Work out the finished part from the listing and answer in its coordinate system (mm). Face numbers are marked on the shaded views. A direction names the side the tool comes from. Coordinates: 2 decimals unless noted, no trailing zeros. Order: outer loops, then holes, each group sorted by start corner. A loop starts at its lowest first (then second) coordinate and runs counter-clockwise, first axis right, second up. Notation, with made-up numbers: (-11.5, -16) -> (16.5, -16) arc R23 ccw to (16.5, 15) -> close; hole circle Ø5 at (30, 9.25). An arc over 180 degrees is marked (long way). Use one line per item in the form item = value.
Autodesk Inventor part; units mm, degrees
ref_plane "Work Plane1" through (1.525, 0, 0) normal (0, 0, 1) x (1, 0, 0)
ref_plane "YZ Plane" through (0, 0, 0) normal (1, 0, 0) x (0, 1, 0)
ref_plane "XZ Plane" through (0, 0, 0) normal (0, 1, 0) x (-1, 0, 0)
sketch "Sketch1" plane through (0, 0, 0) normal (0, 0, 1) x (1, 0, 0)
  line L0 (0, 5.0006) -> (0, 3.175)
  line L1 (3.175, 3.175) -> (19.05, 3.175)
  line L2 (19.05, 3.175) -> (19.05, 0)
  line L3 (19.05, 0) -> (-0.6351, 0)
  line L4 (-4.5721, 0) -> (22.987, 0)
  line L5 (-0.6351, 0) -> (-0.6351, 5.0006)
  line L6 (-0.6351, 5.0006) -> (0, 5.0006)
  line L7 (3.175, 3.175) -> (1.9049, 3.175)
  line L8 (1.9049, 3.175) -> (0, 3.175)
  line L9 (0, -1.0001) -> (0, 6.0007)
  dimension "d0" = 19.05
  dimension "d1" = 15.875
  dimension "d2" = 6.35
  dimension "d9" = 0.6351
  dimension "d10" = 10.0013
  dimension "d13" = 1.2701
  dimension "d14" = 6.35
revolve "Body" add sketch "Sketch1" angle 360 about axis through (19.05, 0, 0) along (-1, 0, 0)
sketch "Sketch2" plane through (-0.6351, 0, 0) normal (-1, 0, 0) x (0, 0, 1)
  line L0 (0, 6.4158) -> (5.5562, 3.2079)
  line L1 (5.5562, 3.2079) -> (5.5562, -3.2079)
  line L2 (5.5562, -3.2079) -> (0, -6.4158)
  line L3 (0, -6.4158) -> (-5.5562, -3.2079)
  line L4 (-5.5562, -3.2079) -> (-5.5562, 3.2079)
  line L5 (-5.5562, 3.2079) -> (0, 6.4158)
  point P0 (0, 0)
  point P1 (0, 0)
  dimension "d11" = 11.1125
extrude "Head" add sketch "Sketch2" along normal blind 3.3337
sketch "Sketch4" plane through (0, 0, 0) normal (0, 0, 1) x (1, 0, 0)
  line L0 (-3.9689, 5.5563) -> (-3.9689, 6.4158)
  line L1 (-3.9689, 6.4158) -> (-3.4726, 6.4158)
  line L2 (-3.4726, 6.4158) -> (-3.9689, 5.5563)
  line L3 (-4.6356, 0) -> (0.0317, 0)
  line L4 (-0.6351, 6.4158) -> (-3.9688, 6.4158)
  line L5 (-3.9688, 3.2079) -> (-3.9688, 6.4158)
  dimension "d5" = 30
  dimension "d19" = 11.1125
revolve "Chamfer1" cut sketch "Sketch4" angle 360 about axis through (-10, 0, 0) along (1, 0, 0)
thread "Thread"
chamfer "Chamfer2" distance 0.6875 distance2 1.2701 1 edges at (19.05, -3.175, 0) measured on face at (19.05, -0.5663, 0.5832)
ref_plane "Work Plane1" through (1.525, 0, 0) normal (0, 0, 1) x (1, 0, 0)
fillet "Fillet2" radius 0.635 1 edges at (0, -3.175, 0)
equation "\"d0\" = NLG"
equation "\"d1\" = GEL"
equation "\"d2\" = GD"
equation "\"d10\" = SD2"
equation "\"d14\" = BDM"
equation "\"d11\" = SW"
equation "\"d3\" = KOH - SD"
equation "\"d5\" = ANG1"
equation "\"d19\" = SW0"
equation "\"d63\" = R"
equation "\"d15\" = GEL"
equation "\"d6\" = -0.5 * SPD + 0.5 * GD"
equation "\"NLG\" = 19.05"
equation "\"GD\" = NND"
equation "\"BDM\" = 6.35"
equation "\"KOH\" = 3.96875"
equation "\"GEL\" = 15.875"
equation "\"SW\" = 11.1125"
equation "\"SW0\" = SW"
equation "\"SPD\" = 4.9751"
equation "\"SD2\" = 10.00125"
equation "\"SD\" = 0.635"
equation "\"ANG1\" = 30deg"
equation "\"GAL\" = 1.27"
equation "\"GUL\" = 1.27"
equation "\"R\" = 0.635"
equation "\"d62\" = -NLG - SD + GUL"
equation "\"THREADDIA\" = 6.35"
equation "\"TOA\" = 30deg"
equation "\"RR\" = 0.254"
equation "\"NND\" = 6.35"
equation "\"E0\" = 1.155 * SW"
equation "\"SLG\" = 0"
equation "\"GD1\" = 4.9751"
properties part number "ANSI B18.2.1 - 1/4-20 UNC - 0.75" material "Steel, Mild"
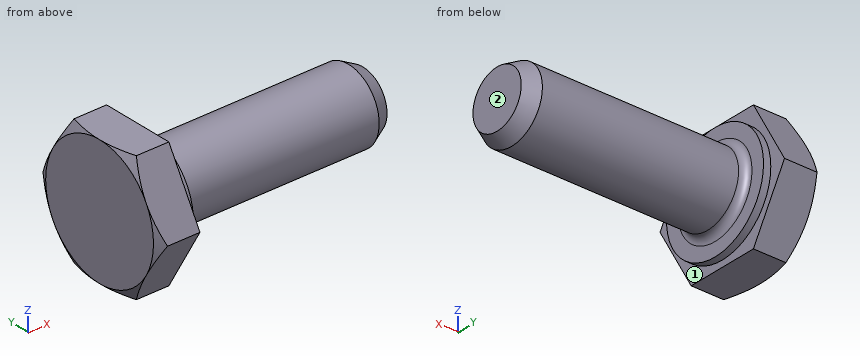
(1) Straight lines are drawn through the part: line 1 along X through (y, z) = (4.75, 1); line 2 along X through (y, z) = (3, 4.25); line 3 along Y through (x, z) = (-2.5, 2.5). For each, find the intervals that lie inside material, in ascending order.
Data:
line_1 = -3.97 to 0
line_2 = -3.97 to -0.64
line_3 = -4.97 to 4.97
(2) Section A-A on x = 5.75 is taken. Write down the section's boundary in (y, z) (3 decimals), plus the area to 3 significant figures.
Data:
outline = circle Ø6.35 at (0, 0)
area = 31.7 mm²
(3) Which of the six approach directions +Z, -Z, +X, -X, +Y, -Y give full straight-line access (tool end or side, diameter ignored) to the marked faces 1 and 2?
Data:
face_1 = +X
face_2 = +Z, -Z, +X, +Y, -Y
(4) Each of these flat-tipped pins is pushed along its axis until it touches: P1, Ø1, axis at x = -1, z = -2, coming from the +Y side; P2, Ø3, axis at x = 6.5, z = 1, coming from the -Y side (3 decimals); P3, Ø2, axis at x = 9.5, z = -3.5, coming from the -Y side. Where does it stop, or does it pass through?
Data:
P1 = 5.55
P2 = -3.175
P3 = -1.96
